```python
from build123d import *

# Parameters (mm, degrees)
F0_W     = 85.5
F0_H     = 30
F0_W_2   = 1.2
F0_H_2   = 4
F1_DEPTH = 4
F2_W     = 89.5
F2_H     = 34
F3_DEPTH = 55
F4_W     = 89.5
F4_H     = 34
F4_W_2   = 33
F4_H_2   = 5
F5_DEPTH = 2
F7_DEPTH = 1.25
F8_W     = 1.2
F8_H     = 4
F9_DEPTH = 0.5


with BuildPart() as f1:
    # F0 (on Right) → F1 (new body)
    with BuildSketch(Plane.YZ):
        Polygon((40.75, 32), (-2, 32), (-2, 30), (-2, 26), (-2, 3), (-2, -1), (-2, -2), (87.5, -2), (87.5, -1), (87.5, 3), (87.5, 26), (87.5, 30), (87.5, 32), (44.75, 32), align=None)
        with Locations((42.75, 15)):
            Rectangle(F0_W, F0_H, mode=Mode.SUBTRACT)
        Polygon((40.75, 33.2), (40.75, 32), (44.75, 32), (44.75, 33.2), (42.75, 33.2), align=None)
        with Locations((-2.6, 28)):
            Rectangle(F0_W_2, F0_H_2)
        with Locations((-2.6, 1)):
            Rectangle(F0_W_2, F0_H_2)
        with Locations((88.1, 28)):
            Rectangle(F0_W_2, F0_H_2)
        with Locations((88.1, 1)):
            Rectangle(F0_W_2, F0_H_2)
    extrude(amount=F1_DEPTH)

    # F2 (on face) → F3 (join)
    with BuildSketch(Plane.YZ.offset(4)):
        with Locations((42.75, 15)):
            Rectangle(F2_W, F2_H)
        Polygon((42.75, 0), (4.75, 0), (4.75, 25), (42.75, 25), (80.75, 25), (80.75, 0), align=None, mode=Mode.SUBTRACT)
    extrude(amount=F3_DEPTH)

    # F4 (on face) → F5 (join)
    with BuildSketch(Plane.YZ.offset(59)):
        with Locations((42.75, 15)):
            Rectangle(F4_W, F4_H)
        with Locations((25.75, 6)):
            Rectangle(F4_W_2, F4_H_2, mode=Mode.SUBTRACT)
        with Locations((59.75, 6)):
            Rectangle(F4_W_2, F4_H_2, mode=Mode.SUBTRACT)
    extrude(amount=F5_DEPTH)

    # F6 (on face) → F7 (join)
    with BuildSketch(Plane(origin=(0, 0, 0), x_dir=(0, -1, 0), z_dir=(-1, 0, 0))):
        Polygon((-87.5, 29.1), (-87.5, 30), (-88.7, 30), (-88.7, 26), (-87.5, 26), (-87.5, 26.9), (-88.15, 26.9), (-88.15, 29.1), align=None)
    extrude(amount=F7_DEPTH)

    # F8 (on face) → F9 (join)
    with BuildSketch(Plane(origin=(-1.25, 0, 0), x_dir=(0, -1, 0), z_dir=(-1, 0, 0))):
        with Locations((-88.1, 28)):
            Rectangle(F8_W, F8_H)
    extrude(amount=F9_DEPTH)


solid = f1.part
```
Design review of the part built by this model. Coordinates are the model's own, in mm. A direction names the side the tool comes from. Coordinates: 2 decimals unless noted, no trailing zeros. Loops run counter-clockwise (first coordinate to the right, second up) from the corner with the lowest first, then second, coordinate; pieces in that order, holes last.
Q1. We need section B-B on z = 28. State the section outline as (x, y) points, and give its area (3 significant figures).
Reported:
outline: (-1.75, 87.5) - (-1.25, 87.5) - (-1.25, 88.15) - (0, 88.15) - (0, 85.5) - (4, 85.5) - (4, 0) - (0, 0) - (0, -3.2) - (4, -3.2) - (4, -2) - (61, -2) - (61, 87.5) - (4, 87.5) - (4, 88.7) - (-1.75, 88.7) - close
area: 5,130 mm2
Q2. Tool access review of faces 1 (the face through (2, 88.7, 1)), 2 (the face through (60, 76.25, 6)), 3 (the face through (29, 43, 0)): name each direction out of +Z, -Z, +X, -X, +Y, -Y from which nothing blocks a thin tool from reaching the whole face with its end or side.
Reported:
face 1: +Z, -Z, +X, -X, +Y
face 2: +X, -X
face 3: -X
Q3. We need section D-D on z = 23.5. State the section outline as (x, y) points, and give its area (4 significant figures).
Reported:
outline: (0, -2) - (61, -2) - (61, 87.5) - (0, 87.5) - (0, 85.5) - (4, 85.5) - (4, 80.75) - (59, 80.75) - (59, 4.75) - (4, 4.75) - (4, 0) - (0, 0) - close
area: 937.5 mm2
Q4. We need section C-C on x = 47.5. State the section outline as (y, z) points.
Reported:
outline: (-2, -2) - (87.5, -2) - (87.5, 32) - (-2, 32) - close; hole (4.75, 0) - (80.75, 0) - (80.75, 25) - (4.75, 25) - close
Q5. For pin 1 (1.5 mm diameter, centred on x = 9, z = 16.5, fed in from -Y); pin 2 (2 mm diameter, centred on x = 52, y = 15, fed in from +Z); pin 3 (1 mm diameter, centred on y = 27.5, z = 13.5, fed in from -X), all flat-tipped, find the tip position at first contact; note any pin that passes through.
Reported:
pin 1: stops at y = -2
pin 2: stops at z = 32
pin 3: stops at x = 59
Q6. We need section A-A on y = 34. State the section outline as (x, z) points, and give its area (3 significant figures).
Reported:
outline: (0, -2) - (61, -2) - (61, 3.5) - (59, 3.5) - (59, 0) - (0, 0) - close; (0, 30) - (4, 30) - (4, 25) - (59, 25) - (59, 8.5) - (61, 8.5) - (61, 32) - (0, 32) - close
area: 569 mm2
Q7. The part is to be moulded in two halves that separate along Y. For faces 4 (the face through (1, 88.7, 28)), 5 (the face through (30, 42, 32)), 6 (the face through (4, 39, 26)), say which applies: +Y half, -Y half, draft (parallel to the pull), parting line (faces both ways), or undercut.
Reported:
face 4: +Y half
face 5: draft
face 6: undercut
Q8. To check wall thickness, follow line 1 (Y direction, x = 56.5, z = 22.5); line 2 (Z direction, x = 6, y = 35); line 3 (X direction, y = 69, z = 9.5). State the ranges of each line that lie inside material, in increasing order.
Reported:
line 1: y = -2 to 4.75, 80.75 to 87.5
line 2: z = -2 to 0, 25 to 32
line 3: x = 59 to 61
